Autodesk Inventor part; units mm, degrees
ref_plane "YZ Plane" through (0, 0, 0) normal (1, 0, 0) x (0, 1, 0)
ref_plane "XZ Plane" through (0, 0, 0) normal (0, 1, 0) x (-1, 0, 0)
ref_plane "XY Plane" through (0, 0, 0) normal (0, 0, 1) x (1, 0, 0)
sketch "Sketch1" plane through (0, 0, 0) normal (0, 1, 0) x (-1, 0, 0)
  circle A0 centre (0, 0) radius 100
  dimension "d0" = 200
extrude "Extrusion1" add sketch "Sketch1" along normal blind 5
sketch "Sketch2" plane through (0, 5, 0) normal (0, 1, 0) x (1, 0, 0)
  circle A0 centre (0, 0) radius 2.5
  circle A1 centre (0, 0) radius 5
  dimension "d3" = 5
  dimension "d4" = 10
extrude "Extrusion2" add sketch "Sketch2" along normal blind 20
fillet "Fillet1" radius 10 1 edges at (-5, 5, 0)
properties part number "podlaga_za_vrtrenje"
Input: part model. Units: mm. Frame: model coordinates. A direction names the side the tool comes from. Round coordinates to 2 decimals unless told otherwise and drop trailing zeros. Loops run counter-clockwise (first coordinate to the right, second up) from the corner with the lowest first, then second, coordinate; pieces in that order, holes last. Notation, with made-up numbers: (46.25, 1) -> (54.25, 1) arc R22 ccw to (54.25, 32) -> close; hole circle Ø9 at (53, 23.25). An arc over 180 degrees is marked (long way). Use one line per item in the form item = value. Start each with the question number.
Item 1: Material intervals for L1, parallel to X at y = 16.5, z = 0; L2, parallel to Z at x = 0, y = 12.75, sorted ascending. Write a range as from..to.
Item 2: Section query D-D on z = -80. Return the cut outline in (x, y), then the cut area to 3 significant figures.
Item 3: Section query B-B on z = 0. Return the cut outline in (x, y).
Item 4: Section query C-C on y = 22. Return the cut outline in (x, z), then the cut area to 3 significant figures.
Item 5: Set-up query: faces 1 (the face through (1, 0, 1)), 2 (the face through (-1.08, 19.93, -4.88)). Return all of +Z, -Z, +X, -X, +Y, -Y with unobstructed straight access to the full face (end or side cutting, diameter ignored); none if empty.
Item 6: Contact query for flat-ended pins moving along their axis: pin 1 Ø4 at (x, z) = (-79, 40.5) entering from -Y; pin 2 Ø4 at (x, y) = (51.5, 4) entering from -Z; pin 3 Ø8 at (y, z) = (6.5, -38.5) entering from +X; pin 4 Ø3 at (x, z) = (-29.5, -66) entering from +Y. Output: stop coordinate, or through.
Item 7: Mould query, pull axis X, two halves, no side actions, for faces 3 (the face through (-95.38, 2.46, -30.04)), 4 (the face through (2, 25, 2)), 5 (the face through (0, 5, 0)). Classes: pulls with the +X half, pulls with the -X half, needs draft (parallel to the pull), parting line crosses it, or undercut.
Item 8: Section query A-A on x = 0. Return the cut outline in (y, z), then the cut area to 3 significant figures.
Ans:
q1.L1 = -5..-2.5, 2.5..5
q1.L2 = -5.26..-2.5, 2.5..5.26
q2.outline = (-60, 0) -> (60, 0) -> (60, 5) -> (-60, 5) -> close
q2.area = 600 mm^2
q3.outline = (-100, 0) -> (100, 0) -> (100, 5) -> (15, 5) arc R10 cw to (5, 15) -> (5, 25) -> (2.5, 25) -> (2.5, 5) -> (-2.5, 5) -> (-2.5, 25) -> (-5, 25) -> (-5, 15) arc R10 cw to (-15, 5) -> (-100, 5) -> close
q4.outline = circle Ø10 at (0, 0); hole circle Ø5 at (0, 0)
q4.area = 58.9 mm^2
q5.face_1 = +Z, -Z, +X, -X, -Y
q5.face_2 = +Y
q6.pin_1 = 0
q6.pin_2 = -86.89
q6.pin_3 = 93.75
q6.pin_4 = 5
q7.face_3 = parting line crosses it
q7.face_4 = needs draft
q7.face_5 = undercut
q8.outline = (0, -100) -> (5, -100) -> (5, -15) arc R10 cw to (15, -5) -> (25, -5) -> (25, -2.5) -> (5, -2.5) -> (5, 2.5) -> (25, 2.5) -> (25, 5) -> (15, 5) arc R10 cw to (5, 15) -> (5, 100) -> (0, 100) -> close
q8.area = 1,140 mm^2
